The model under review builds one solid part; all positions refer to its coordinate system, in mm. Face numbers are marked on the shaded views. A direction names the side the tool comes from. Coordinates: 2 decimals unless noted, no trailing zeros. Order: outer loops, then holes, each group sorted by start corner. A loop starts at its lowest first (then second) coordinate and runs counter-clockwise, first axis right, second up.
from build123d import *

# Parameters (mm, degrees)
F0_R      = 2.5
F1_DEPTH  = 30
F2_DEPTH  = 5
F3_DEPTH  = 5
F4_R      = 1
F5_DEPTH  = 5
F7_DEPTH  = 23
F8_DEPTH  = 4
F9_R      = 1
F10_DEPTH = 5
F11_R     = 1
F12_DEPTH = 5


# Not quite as in the source:
# - a pattern or mirror of a feature is missing from the dataset's text; its kind, count and spacing are read off the source's solid


with BuildPart() as f1:
    # F0 (on Front) → F1 (new body)
    with BuildSketch(Plane.XZ):
        with BuildLine():
            Line((14.7980262304, 19.5), (-22.7980262304, 19.5))
            ThreePointArc((-22.7980262304, 19.5), (-30, 0), (-22.7980262304, -19.5))
            Line((-22.7980262304, -19.5), (14.7980262304, -19.5))
            ThreePointArc((14.7980262304, -19.5), (22, 0), (14.7980262304, 19.5))
        make_face()
        with BuildLine():
            ThreePointArc((-17.1245437895, 7), (3.5669272416, 18.1528793874), (18.5, 0))
            ThreePointArc((18.5, 0), (1.5049882267, -18.4386824485), (-18.2551362635, -3))
            Line((-18.2551362635, -3), (-19.5, -3))
            ThreePointArc((-19.5, -3), (-24.5, 2), (-19.5, 7))
            Line((-19.5, 7), (-17.1245437895, 7))
        make_face(mode=Mode.SUBTRACT)
        with BuildLine():
            ThreePointArc((-18.2551362635, -3), (1.5049882267, -18.4386824485), (18.5, 0))
            ThreePointArc((18.5, 0), (3.5669272416, 18.1528793874), (-17.1245437895, 7))
            ThreePointArc((-17.1245437895, 7), (-17.2243437117, 6.7507024597), (-17.320514605, 6.4999826014))
            ThreePointArc((-17.320514605, 6.4999826014), (-15.2634077978, 4.6554258627), (-14.5, 2))
            ThreePointArc((-14.5, 2), (-15.5564468025, -1.0738230558), (-18.2793552714, -2.8487138961))
            ThreePointArc((-18.2793552714, -2.8487138961), (-18.2674023824, -2.9243820202), (-18.2551362635, -3))
        make_face()
        Circle(F0_R, mode=Mode.SUBTRACT)
        with BuildLine():
            ThreePointArc((-18.2793552714, -2.8487138961), (-18.4034566143, 1.8875340117), (-17.320514605, 6.4999826014))
            ThreePointArc((-17.320514605, 6.4999826014), (-18.3819465592, 6.8733927098), (-19.5, 7))
            ThreePointArc((-19.5, 7), (-24.5, 2), (-19.5, -3))
            ThreePointArc((-19.5, -3), (-18.885007919, -2.9620343349), (-18.2793552714, -2.8487138961))
        make_face()
        with BuildLine():
            ThreePointArc((-14.5, 2), (-15.2634077978, 4.6554258627), (-17.320514605, 6.4999826014))
            ThreePointArc((-17.320514605, 6.4999826014), (-18.4034566143, 1.8875340117), (-18.2793552714, -2.8487138961))
            ThreePointArc((-18.2793552714, -2.8487138961), (-15.5564468025, -1.0738230558), (-14.5, 2))
        make_face()
        with BuildLine():
            ThreePointArc((-17.320514605, 6.4999826014), (-17.2243437117, 6.7507024597), (-17.1245437895, 7))
            Line((-17.1245437895, 7), (-19.5, 7))
            ThreePointArc((-19.5, 7), (-18.3819465592, 6.8733927098), (-17.320514605, 6.4999826014))
        make_face()
        with BuildLine():
            Line((-19.5, -3), (-18.2551362635, -3))
            ThreePointArc((-18.2551362635, -3), (-18.2674023824, -2.9243820202), (-18.2793552714, -2.8487138961))
            ThreePointArc((-18.2793552714, -2.8487138961), (-18.885007919, -2.9620343349), (-19.5, -3))
        make_face()
        Circle(F0_R)
    extrude(amount=-F1_DEPTH)

    # F0 (on Front) → F2 (cut)
    with BuildSketch(Plane.XZ):
        with BuildLine():
            ThreePointArc((-18.2551362635, -3), (1.5049882267, -18.4386824485), (18.5, 0))
            ThreePointArc((18.5, 0), (3.5669272416, 18.1528793874), (-17.1245437895, 7))
            ThreePointArc((-17.1245437895, 7), (-17.2243437117, 6.7507024597), (-17.320514605, 6.4999826014))
            ThreePointArc((-17.320514605, 6.4999826014), (-15.2634077978, 4.6554258627), (-14.5, 2))
            ThreePointArc((-14.5, 2), (-15.5564468025, -1.0738230558), (-18.2793552714, -2.8487138961))
            ThreePointArc((-18.2793552714, -2.8487138961), (-18.2674023824, -2.9243820202), (-18.2551362635, -3))
        make_face()
        Circle(F0_R, mode=Mode.SUBTRACT)
        with BuildLine():
            ThreePointArc((-17.320514605, 6.4999826014), (-17.2243437117, 6.7507024597), (-17.1245437895, 7))
            Line((-17.1245437895, 7), (-19.5, 7))
            ThreePointArc((-19.5, 7), (-18.3819465592, 6.8733927098), (-17.320514605, 6.4999826014))
        make_face()
        with BuildLine():
            Line((-19.5, -3), (-18.2551362635, -3))
            ThreePointArc((-18.2551362635, -3), (-18.2674023824, -2.9243820202), (-18.2793552714, -2.8487138961))
            ThreePointArc((-18.2793552714, -2.8487138961), (-18.885007919, -2.9620343349), (-19.5, -3))
        make_face()
        with BuildLine():
            ThreePointArc((-18.2793552714, -2.8487138961), (-18.4034566143, 1.8875340117), (-17.320514605, 6.4999826014))
            ThreePointArc((-17.320514605, 6.4999826014), (-18.3819465592, 6.8733927098), (-19.5, 7))
            ThreePointArc((-19.5, 7), (-24.5, 2), (-19.5, -3))
            ThreePointArc((-19.5, -3), (-18.885007919, -2.9620343349), (-18.2793552714, -2.8487138961))
        make_face()
        with BuildLine():
            ThreePointArc((-14.5, 2), (-15.2634077978, 4.6554258627), (-17.320514605, 6.4999826014))
            ThreePointArc((-17.320514605, 6.4999826014), (-18.4034566143, 1.8875340117), (-18.2793552714, -2.8487138961))
            ThreePointArc((-18.2793552714, -2.8487138961), (-15.5564468025, -1.0738230558), (-14.5, 2))
        make_face()
    extrude(amount=-F2_DEPTH, mode=Mode.SUBTRACT)

    # F0 (on Front) → F3 (join)
    with BuildSketch(Plane.XZ):
        Circle(F0_R)
    extrude(amount=F3_DEPTH)

    # F4 (on face) → F5 (cut)
    with BuildSketch(Plane.XY.offset(19.5)):
        with Locations((-11.5, 15)):
            Circle(F4_R)
        with Locations((3, 15)):
            Circle(F4_R)
    f5 = extrude(amount=-F5_DEPTH, mode=Mode.SUBTRACT)

    # F5_copies: F5 across plane
    add(f5.mirror(Plane(origin=(0, 0, 0), x_dir=(-1, 0, 0), z_dir=(0, 0, -1))), mode=Mode.SUBTRACT)

    # F6 (on face) → F7 (join)
    with BuildSketch(Plane(origin=(0, 30, 0), x_dir=(-1, 0, 0), z_dir=(0, 1, 0))):
        with BuildLine():
            Line((-27, -16.5), (-17.0549396327, -16.5))
            ThreePointArc((-17.0549396327, -16.5), (-21.5046036204, -5.4293982359), (-21.2873692912, 6.5))
            Line((-21.2873692912, 6.5), (-27, 6.5))
            Line((-27, 6.5), (-27, -16.5))
        make_face()
    extrude(amount=-F7_DEPTH)

    # F6 (on face) → F8 (join)
    with BuildSketch(Plane(origin=(0, 30, 0), x_dir=(-1, 0, 0), z_dir=(0, 1, 0))):
        with BuildLine():
            ThreePointArc((0, 2.5), (-2.5, 0), (0, -2.5))
            Line((0, -2.5), (0, 2.5))
        make_face()
        with BuildLine():
            Line((0, 2.5), (0, -2.5))
            ThreePointArc((0, -2.5), (1.767766953, -1.767766953), (2.5, 0))
            ThreePointArc((2.5, 0), (1.767766953, 1.767766953), (0, 2.5))
        make_face()
    extrude(amount=F8_DEPTH)

    # F9 (on face) → F10 (cut)
    with BuildSketch(Plane.XZ.offset(5)):
        Circle(F9_R)
    extrude(amount=-F10_DEPTH, mode=Mode.SUBTRACT)

    # F11 (on face) → F12 (cut)
    with BuildSketch(Plane(origin=(0, 34, 0), x_dir=(-1, 0, 0), z_dir=(0, 1, 0))):
        Circle(F11_R)
    extrude(amount=-F12_DEPTH, mode=Mode.SUBTRACT)


solid = f1.part
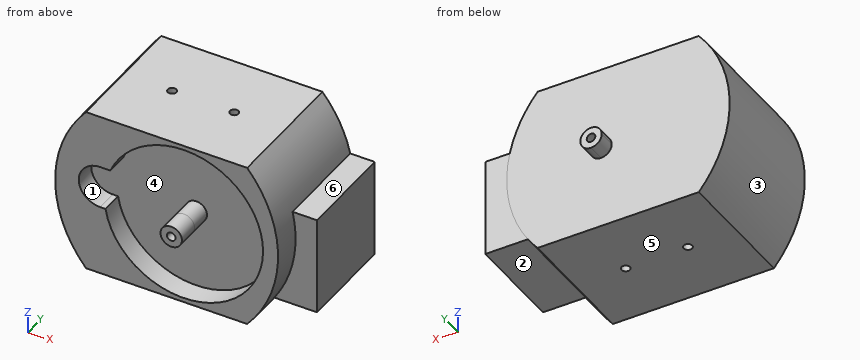
(1) Insertion check: pin 1 Ø3 at (x, z) = (12, 6.5) entering from -Y; pin 2 Ø1 at (x, y) = (3, 15) entering from +Z; pin 3 Ø5 at (x, z) = (-9.5, -4.5) entering from +Y. Each pin has a flat end and moves straight along its axis. Give the tip position at first contact, or say it passes through.
(2) Tool access review of the marked faces 1, 2 and 3: name each direction out of +Z, -Z, +X, -X, +Y, -Y from which nothing blocks a thin tool from reaching the whole face with its end or side.
(3) Consider section D-D (x = 7.5). Give the boundary of the cut face in (y, z), then the cut area to 3 significant figures.
(4) Wall thickness on line 1 (Y direction, x = 3, z = 17.15); line 2 (Y direction, x = -11.5, z = 17.25); line 3 (Y direction, x = 19, z = -7): over which ranges is each line inside the solid? List them lowest first.
(5) Consider section C-C (x = -11.5). Give the boundary of the cut face in (y, z).
(6) The part is to be moulded in two halves that separate along Z. For the marked faces 4, 5 and 6, say which applies: +Z half, -Z half, draft (parallel to the pull), parting line (faces both ways), or undercut.
(7) Consider section B-B (z = 4). Give the boundary of the cut face in (x, y).
(8) Consider section A-A (y = 17.5). Give the boundary of the cut face in (x, z).
Findings:
1. pin 1: stops at y = 5
1. pin 2: stops at z = 14.5
1. pin 3: stops at y = 30
2. face 1: -Y
2. face 2: -Z, +X, +Y, -Y
2. face 3: -X, +Y, -Y
3. outline: (0, -19.5) - (30, -19.5) - (30, 19.5) - (0, 19.5) - (0, 16.91) - (5, 16.91) - (5, -16.91) - (0, -16.91) - close
3. area: 1,000 mm2
4. line 1: y = 5 to 14, 16 to 30
4. line 2: y = 0 to 14, 16 to 30
4. line 3: y = 0 to 30
5. outline: (0, -19.5) - (14, -19.5) - (14, -14.5) - (16, -14.5) - (16, -19.5) - (30, -19.5) - (30, 19.5) - (16, 19.5) - (16, 14.5) - (14, 14.5) - (14, 19.5) - (0, 19.5) - (0, 14.49) - (5, 14.49) - (5, -14.49) - (0, -14.49) - close
6. face 4: undercut
6. face 5: -Z half
6. face 6: +Z half
7. outline: (-29.73, 0) - (-24.08, 0) - (-24.08, 5) - (18.06, 5) - (18.06, 0) - (21.73, 0) - (21.73, 7) - (27, 7) - (27, 30) - (-29.73, 30) - close
8. outline: (-22.8, -19.5) - (14.8, -19.5) arc R30 ccw to (17.05, -16.5) - (27, -16.5) - (27, 6.5) - (21.29, 6.5) arc R30 ccw to (14.8, 19.5) - (-22.8, 19.5) arc R30 ccw to start
